Read the model definition and answer for the solid it produces. Units are mm, in the model's axes. A direction names the side the tool comes from. Coordinates: 2 decimals unless noted, no trailing zeros. Order: outer loops, then holes, each group sorted by start corner. A loop starts at its lowest first (then second) coordinate and runs counter-clockwise, first axis right, second up. Notation, with made-up numbers: (-5, 31.5) -> (16, 31.5) arc R9 ccw to (16, 47.5) -> close; hole circle Ø4 at (-21, 31). An arc over 180 degrees is marked (long way). Answer as a JSON object with one key per item and string values. Group by question number.
1) Section C-C on x = 8 is taken. Determine the outline of the cut face in (y, z), and give its area (3 significant figures).
2) Consider L1, parallel to Y at x = 0, z = -1.85; L2, parallel to Y at x = 19.05, z = -0.8 (3 decimals); L3, parallel to X at y = 2, z = -1.5. Determine where each line is inside the solid, lowest interval first.
3) Determine the mould class of faces 1 (the flat face through (9.791, -3.947, 0.783)), 2 (the flat face through (10, -0.397, -1)), 3 (the flat face through (11, 0, 1.588)) for opening direction X: released by +X, released by -X, zero draft, split by the parting line, or undercut.
4) Given pin 1 (2 mm diameter, centred on x = 13, y = 0, fed in from -Z); pin 2 (1 mm diameter, centred on x = 19.05, y = 0, fed in from -Z); pin 3 (5 mm diameter, centred on x = 4, z = 0, fed in from +Y); pin 4 (1 mm diameter, centred on x = 10.5, z = -1, fed in from -Y), each flat-ended and moving along its own axis, determine where each tip first touches the part or whether it passes through.
5) Section D-D on y = 3.5 is taken. Determine the outline of the cut face in (x, z).
6) Section B-B on x = -0.75 is taken. Determine the outline of the cut face in (y, z), and give its area (3 significant figures).
7) Section A-A on z = 1.25 is taken. Count the separate pieces of the cut face and the enclosed holes in it, and give its area (3 significant figures).
8) A tool of negligible diameter and unlimited length cuts with its end or side. For faces 4 (the flat face through (10.24, 0.01, -2.68)), 5 (the flat face through (10, 2, 0)), 6 (the flat face through (10, -2, 0)), from which of +Z, -Z, +X, -X, +Y, -Y can it reach the whole face along a straight path? Write none if from no direction.
from build123d import *
from build123d import SkipClean  # not in build123d's __all__

# Parameters (mm, degrees)
F1_DEPTH  = 1.5875
F2_R      = 4.7625
F2_R_2    = 2.38125
F3_DEPTH  = 3.175
F4_R      = 4.7625
F4_R_2    = 2.38125
F5_DEPTH  = 3.96875
F6_R      = 3.175
F6_R_2    = 0.79375
F7_DEPTH  = 2.38125
F9_DEPTH  = 3.96875
F11_DEPTH = 25.4


with BuildPart() as f1:
    # F0 (on Top) → F1 (new body)
    with BuildSketch(Plane.XY):
        with BuildLine():
            Line((0.7882758621, 4.6968103448), (0, 4.7625))
            ThreePointArc((0, 4.7625), (-4.7625, 0), (0, -4.7625))
            Line((0, -4.7625), (0.7882758621, -4.6968103448))
            ThreePointArc((0.7882758621, -4.6968103448), (3.6356271841, -3.076299925), (4.7625, 0))
            ThreePointArc((4.7625, 0), (3.6356271841, 3.076299925), (0.7882758621, 4.6968103448))
        make_face()
        with BuildLine():
            ThreePointArc((2.38125, 0), (1.6837980227, -1.6837980227), (0, -2.38125))
            ThreePointArc((0, -2.38125), (-1.6837980227, 1.6837980227), (2.38125, 0))
        make_face(mode=Mode.SUBTRACT)
        with BuildLine():
            ThreePointArc((0.7882758621, 4.6968103448), (0.3955040978, 4.7460491736), (0, 4.7625))
            Line((0, 4.7625), (0.7882758621, 4.6968103448))
        make_face()
        with BuildLine():
            Line((0.7882758621, -4.6968103448), (0, -4.7625))
            ThreePointArc((0, -4.7625), (0.3955040978, -4.7460491736), (0.7882758621, -4.6968103448))
        make_face()
        with BuildLine():
            Line((19.05, 3.175), (0.7882758621, 4.6968103448))
            ThreePointArc((0.7882758621, 4.6968103448), (3.6356271841, 3.076299925), (4.7625, 0))
            ThreePointArc((4.7625, 0), (3.6356271841, -3.076299925), (0.7882758621, -4.6968103448))
            Line((0.7882758621, -4.6968103448), (19.05, -3.175))
            ThreePointArc((19.05, -3.175), (15.875, 0), (19.05, 3.175))
        make_face()
        with BuildLine():
            ThreePointArc((22.225, 0), (21.2950640303, 2.2450640303), (19.05, 3.175))
            ThreePointArc((19.05, 3.175), (15.875, 0), (19.05, -3.175))
            ThreePointArc((19.05, -3.175), (21.2950640303, -2.2450640303), (22.225, 0))
        make_face()
        with BuildLine():
            ThreePointArc((19.84375, 0), (19.6112660076, -0.5612660076), (19.05, -0.79375))
            ThreePointArc((19.05, -0.79375), (18.4887339924, 0.5612660076), (19.84375, 0))
        make_face(mode=Mode.SUBTRACT)
    extrude(amount=F1_DEPTH)

    # F2 (on face) → F3 (join)
    with BuildSketch(Plane.XY.offset(1.5875)):
        Circle(F2_R)
        Circle(F2_R_2, mode=Mode.SUBTRACT)
    with SkipClean():  # cleaning this boolean's faces spoils the solid; the shape is the same uncleaned
        extrude(amount=F3_DEPTH)

    # F4 (on face) → F5 (join)
    with BuildSketch(Plane(origin=(0, 0, 0), x_dir=(1, 0, 0), z_dir=(0, 0, -1))):
        Circle(F4_R)
        Circle(F4_R_2, mode=Mode.SUBTRACT)
    extrude(amount=F5_DEPTH)

    # F6 (on face) → F7 (join)
    with BuildSketch(Plane(origin=(0, 0, 0), x_dir=(1, 0, 0), z_dir=(0, 0, -1))):
        with Locations((19.05, 0)):
            Circle(F6_R)
        with Locations((19.05, 0)):
            Circle(F6_R_2, mode=Mode.SUBTRACT)
    extrude(amount=F7_DEPTH)

    # F8 (on face) → F9 (join, through all)
    with BuildSketch(Plane(origin=(0, 0, -3.96875), x_dir=(1, 0, 0), z_dir=(0, 0, -1))):
        with BuildLine():
            ThreePointArc((4.7459347324, 0.396875), (4.758356881, 0.1986102803), (4.7625, 0))
            ThreePointArc((4.7625, 0), (4.758356881, -0.1986102803), (4.7459347324, -0.396875))
            Line((4.7459347324, -0.396875), (15.8999023453, -0.396875))
            ThreePointArc((15.8999023453, -0.396875), (15.875, 0), (15.8999023453, 0.396875))
            Line((15.8999023453, 0.396875), (4.7459347324, 0.396875))
        make_face()
    extrude(amount=-F9_DEPTH)

    # F10 (on face) → F11 (cut)
    with BuildSketch(Plane(origin=(0, 0.396875, 0), x_dir=(-1, 0, 0), z_dir=(0, 1, 0))):
        Polygon((-4.7459347324, -3.96875), (-4.7459347324, -3.46075), (-15.8999023453, -1.87325), (-15.8999023453, -2.38125), (-15.8999023453, -3.96875), align=None)
    extrude(amount=-F11_DEPTH, mode=Mode.SUBTRACT)


solid = f1.part
Worked answers:
{
 "1": {"outline": "(-4.1, 0) -> (-0.4, 0) -> (-0.4, -3) -> (0.4, -3) -> (0.4, 0) -> (4.1, 0) -> (4.1, 1.59) -> (-4.1, 1.59) -> close", "area": "15.4 mm²"},
 "2": {"L1": "y = -4.76 to -2.38, 2.38 to 4.76", "L2": "y = -3.175 to -0.794, 0.794 to 3.175", "L3": "x = -4.32 to -1.29, 1.29 to 4.32, 16.58 to 21.52"},
 "3": {"face 1": "released by +X", "face 2": "undercut", "face 3": "zero draft"},
 "4": {"pin 1": "stops at z = -2.43", "pin 2": "passes through", "pin 3": "stops at y = 4.64", "pin 4": "stops at y = -0.4"},
 "5": {"outline": "(-3.23, -3.97) -> (3.23, -3.97) -> (3.23, 0) -> (15.15, 0) -> (15.15, 1.59) -> (3.23, 1.59) -> (3.23, 4.76) -> (-3.23, 4.76) -> close"},
 "6": {"outline": "(-4.7, -3.97) -> (-2.26, -3.97) -> (-2.26, 4.76) -> (-4.7, 4.76) -> close; (2.26, -3.97) -> (4.7, -3.97) -> (4.7, 4.76) -> (2.26, 4.76) -> close", "area": "42.7 mm²"},
 "7": {"separate pieces": "1", "enclosed holes": "2", "area": "183 mm²"},
 "8": {"face 4": "-Z, +Y, -Y", "face 5": "-Z, +Y", "face 6": "-Z, -Y"}
}
